Print and shaded views of the part. All mm, measured from the part's lowest x, y and z. A direction names the side the tool comes from. Coordinates: 2 decimals unless noted, no trailing zeros. Order: outer loops, then holes, each group sorted by start corner. A loop starts at its lowest first (then second) coordinate and runs counter-clockwise, first axis right, second up.
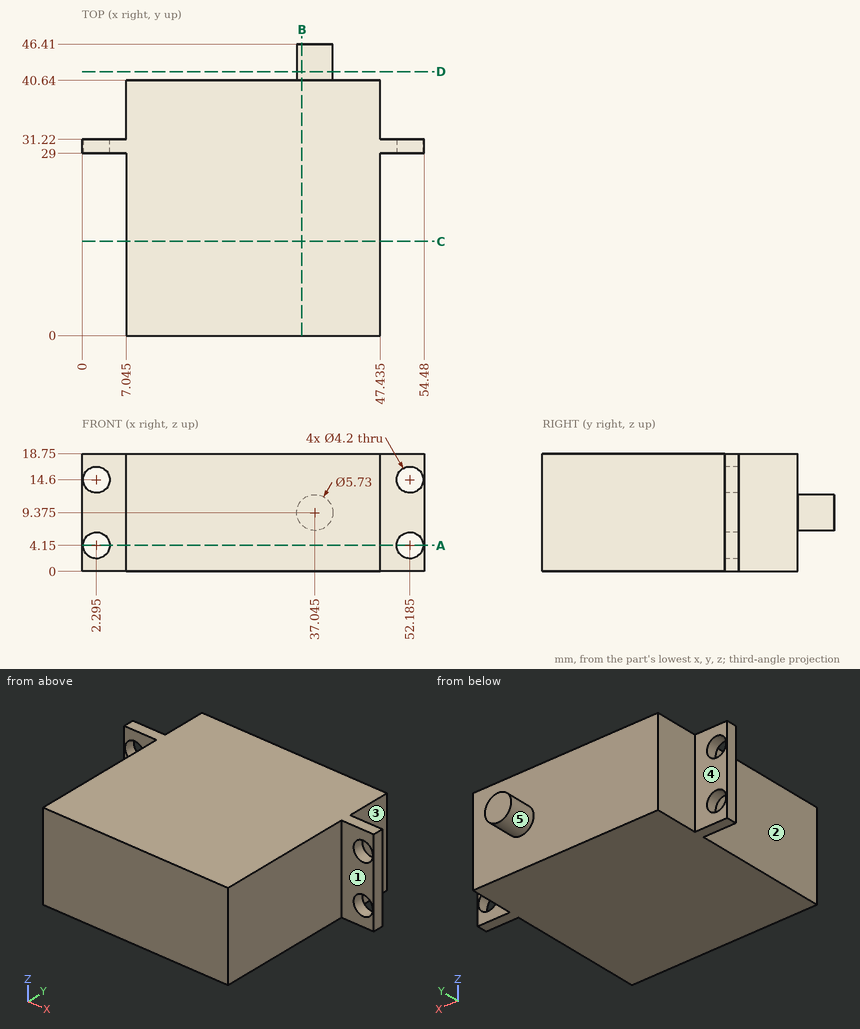
Q1. Which spindle directions (+Z, -Z, +X, -X, +Y, -Y) get a long thin tool onto all of the face, cutting with end or side? Do the marked faces 1, 2, 3, 4 and 5. Say none if no direction does.
Established:
face 1: +Z, -Z, +X, -Y
face 2: +Z, -Z, -X, -Y
face 3: +Z, -Z, +X, +Y
face 4: +Z, -Z, -X, +Y
face 5: +Y
Q2. Probe line 1 (X direction, y = 30.65, z = 14.6) (3 decimals); line 2 (Y direction, x = 33, z = 15.75); line 3 (X direction, y = 19.5, z = 10) (3 decimals). List the from-to ranges inside material, lowest first.
Established:
line 1: x = 0 to 0.195, 4.395 to 50.085, 54.285 to 54.48
line 2: y = 0 to 40.64
line 3: x = 7.045 to 47.435
Q3. Cut at B-B, the plane x = 35. List the corners of the cut face in (y, z), plus the area to 3 significant figures.
Established:
outline: (0, 0) - (40.64, 0) - (40.64, 7.37) - (46.41, 7.37) - (46.41, 11.38) - (40.64, 11.38) - (40.64, 18.75) - (0, 18.75) - close
area: 785 mm2
Q4. Cut at D-D, the plane y = 42. List the corners of the cut face in (x, z) (3 decimals), plus the area to 3 significant figures.
Established:
outline: circle Ø5.73 at (37.045, 9.375)
area: 25.8 mm2
Q5. Cut at A-A, the plane z = 4.15. List the corners of the cut face in (x, y) (3 decimals).
Established:
outline: (0, 29) - (0.195, 29) - (0.195, 31.22) - (0, 31.22) - close; (4.395, 29) - (7.045, 29) - (7.045, 0) - (47.435, 0) - (47.435, 29) - (50.085, 29) - (50.085, 31.22) - (47.435, 31.22) - (47.435, 40.64) - (7.045, 40.64) - (7.045, 31.22) - (4.395, 31.22) - close; (54.285, 29) - (54.48, 29) - (54.48, 31.22) - (54.285, 31.22) - close
Q6. Drop flat-ended pins along their axis: P1, Ø5, axis at x = 45, z = 2, coming from the +Y side; P2, Ø5.5, axis at x = 52.185, z = 14.6, coming from the -Y side; P3, Ø1.5, axis at y = 15.5, z = 15.5, coming from the -X side (3 decimals); P4, Ø4, axis at x = 52.185, z = 4.15, coming from the -Y side. Give the stop position or say it passes through.
Established:
P1: stops at y = 40.64
P2: stops at y = 29
P3: stops at x = 7.045
P4: passes through
Q7. Cut at C-C, the plane y = 15. List the corners of the cut face in (x, z) (3 decimals), plus the area to 3 significant figures.
Established:
outline: (7.045, 0) - (47.435, 0) - (47.435, 18.75) - (7.045, 18.75) - close
area: 757 mm2
